Autodesk Fusion 360 part; units mm, degrees
sketch "Sketch1" plane through (0, 0, 0) normal (0, 0, 1) x (1, 0, 0)
  line L0 (0, 0) -> (76, 0)
  line L1 (76, 0) -> (76, 84)
  line L2 (76, 84) -> (0, 84)
  line L3 (0, 84) -> (0, 0)
  dimension "d1" = 76
  dimension "d2" = 84
extrude "Extrude1" add sketch "Sketch1" along normal blind 2.5
sketch "Sketch2" plane through (0, 0, 2.5) normal (0, 0, 1) x (-1, 0, 0)
  line L0 (0, -84) -> (0, 0)
  line L1 (0, 0) -> (-76, 0)
  line L2 (-76, 0) -> (-76, -84)
  line L3 (-76, -84) -> (0, -84)
  line L4 (0, -84) -> (-4, -84)
  line L5 (-4, -84) -> (-6, -84)
  line L6 (-6, -84) -> (-6, -69)
  line L7 (-6, -69) -> (-4, -69)
  line L8 (-4, -69) -> (-4, -84)
  line L9 (-4, -69) -> (-4, -51)
  line L10 (-4, -51) -> (-6, -51)
  line L11 (-6, -51) -> (-6, -33)
  line L12 (-6, -33) -> (-4, -33)
  line L13 (-4, -33) -> (-4, -51)
  line L14 (-4, -33) -> (-4, -15)
  line L15 (-4, -15) -> (-6, -15)
  line L16 (-6, -15) -> (-6, 0)
  line L17 (-6, 0) -> (-4, 0)
  line L18 (-4, 0) -> (-4, -15)
  line L19 (-6, -84) -> (-40, -84)
  line L20 (-4, -84) -> (-38, -84)
  line L21 (-38, -84) -> (-38, -65)
  line L22 (-72, -69) -> (-72, -84)
  line L23 (-70, -84) -> (-70, -69)
  line L24 (-72, -84) -> (-38, -84)
  line L25 (-70, -69) -> (-72, -69)
  line L26 (-72, -51) -> (-70, -51)
  line L27 (-70, -51) -> (-70, -33)
  line L28 (-72, -33) -> (-72, -51)
  line L29 (-70, -33) -> (-72, -33)
  line L30 (-72, -15) -> (-70, -15)
  line L31 (-70, -15) -> (-70, 0)
  line L32 (-72, 0) -> (-72, -15)
  line L33 (-70, 0) -> (-72, 0)
  dimension "d5" = 4
  dimension "d6" = 2
  dimension "d7" = 15
  dimension "d8" = 18
  dimension "d9" = 2
  dimension "d10" = 18
  dimension "d11" = 18
  dimension "d12" = 2
  dimension "d13" = 15
  dimension "d15" = 34
extrude "Extrude2" add sketch "Sketch2" along normal blind 3 contours L3 L5 L6 L7 L8 L20 | L1 L15 L16 L17 L18 | L10 L11 L12 L13 | L1 L30 L31 L32 L33 | L3 L22 L23 L24 L25 | L26 L27 L28 L29
sketch "Sketch3" plane through (0, 0, 2.5) normal (0, 0, 1) x (-1, 0, 0)
  line L0 (-72, -15) -> (-72, 0)
  line L1 (-72, 0) -> (-76, 0)
  line L2 (-76, 0) -> (-76, -84)
  line L3 (-76, -84) -> (-72, -84)
  line L4 (-72, -84) -> (-72, -69)
  line L5 (-72, -69) -> (-70, -69)
  line L6 (-70, -69) -> (-70, -84)
  line L7 (-70, -84) -> (-6, -84)
  line L8 (-6, -84) -> (-6, -69)
  line L9 (-6, -69) -> (-4, -69)
  line L10 (-4, -69) -> (-4, -84)
  line L11 (-4, -84) -> (0, -84)
  line L12 (0, -84) -> (0, 0)
  line L13 (0, 0) -> (-4, 0)
  line L14 (-4, 0) -> (-4, -15)
  line L15 (-4, -15) -> (-6, -15)
  line L16 (-6, -15) -> (-6, 0)
  line L17 (-6, 0) -> (-70, 0)
  line L18 (-70, 0) -> (-70, -15)
  line L19 (-70, -15) -> (-72, -15)
  line L20 (-4, -33) -> (-4, -51)
  line L21 (-4, -51) -> (-6, -51)
  line L22 (-6, -51) -> (-6, -33)
  line L23 (-6, -33) -> (-4, -33)
  line L24 (-70, -33) -> (-70, -51)
  line L25 (-70, -51) -> (-72, -51)
  line L26 (-72, -51) -> (-72, -33)
  line L27 (-72, -33) -> (-70, -33)
  line L28 (-70, -84) -> (-67.5, -84)
  line L29 (-67.5, -84) -> (-67.5, -79)
  line L30 (-67.5, -79) -> (-55.5, -79)
  line L31 (-55.5, -79) -> (-55.5, -77)
  line L32 (-55.5, -77) -> (-67.5, -77)
  line L33 (-67.5, -77) -> (-67.5, -79)
  line L34 (-67.5, -77) -> (-65.5, -77)
  line L35 (-65.5, -77) -> (-65.5, -67)
  line L36 (-65.5, -67) -> (-67.5, -67)
  line L37 (-67.5, -67) -> (-67.5, -77)
  line L38 (-67.5, -79) -> (-8.5, -79)
  line L39 (-8.5, -79) -> (-8.5, -76)
  line L40 (-8.5, -76) -> (-13.5, -76)
  line L41 (-13.5, -76) -> (-13.5, -74)
  line L42 (-13.5, -74) -> (-8.5, -74)
  line L43 (-8.5, -74) -> (-8.5, -76)
  line L44 (-8.5, -74) -> (-10.5, -74)
  line L45 (-10.5, -74) -> (-10.5, -64)
  line L46 (-10.5, -64) -> (-8.5, -64)
  line L47 (-8.5, -64) -> (-8.5, -74)
  line L48 (-67.5, -67) -> (-67.5, -16)
  line L49 (-67.5, -16) -> (-65.5, -16)
  line L50 (-65.5, -16) -> (-65.5, -6)
  line L51 (-65.5, -6) -> (-67.5, -6)
  line L52 (-67.5, -6) -> (-67.5, -16)
  line L53 (-65.5, -6) -> (-45.5, -6)
  line L54 (-45.5, -6) -> (-35.5, -6)
  line L55 (-35.5, -6) -> (-35.5, -8)
  line L56 (-35.5, -8) -> (-45.5, -8)
  line L57 (-45.5, -8) -> (-45.5, -6)
  line L58 (-35.5, -6) -> (-15.5, -6)
  line L59 (-15.5, -6) -> (-8.5, -6)
  line L60 (-8.5, -6) -> (-8.5, -8)
  line L61 (-8.5, -8) -> (-15.5, -8)
  line L62 (-15.5, -8) -> (-15.5, -6)
  line L63 (-8.5, -8) -> (-10.5, -8)
  line L64 (-10.5, -8) -> (-10.5, -18)
  line L65 (-10.5, -18) -> (-8.5, -18)
  line L66 (-8.5, -18) -> (-8.5, -8)
  dimension "d19" = 2.5
  dimension "d20" = 5
  dimension "d21" = 12
  dimension "d22" = 2
  dimension "d23" = 2
  dimension "d24" = 10
  dimension "d25" = 59
  dimension "d26" = 3
  dimension "d27" = 5
  dimension "d28" = 2
  dimension "d29" = 10
  dimension "d30" = 51
  dimension "d31" = 2
  dimension "d32" = 10
  dimension "d33" = 20
  dimension "d34" = 10
  dimension "d35" = 2
  dimension "d36" = 20
  dimension "d37" = 7
  dimension "d38" = 2
  dimension "d39" = 2
  dimension "d40" = 10
extrude "Extrude3" add sketch "Sketch3" along normal blind 5 contours L59 L60 L61 L62 L63 | L54 L55 L56 L57 | L49 L50 L51 L52 | L40 L41 L42 L43 L44 | L30 L31 L32 L33 L34 L38 | L32 L34 L35 L36 L37 | L42 L44 L45 L46 L47 | L61 L63 L64 L65 L66
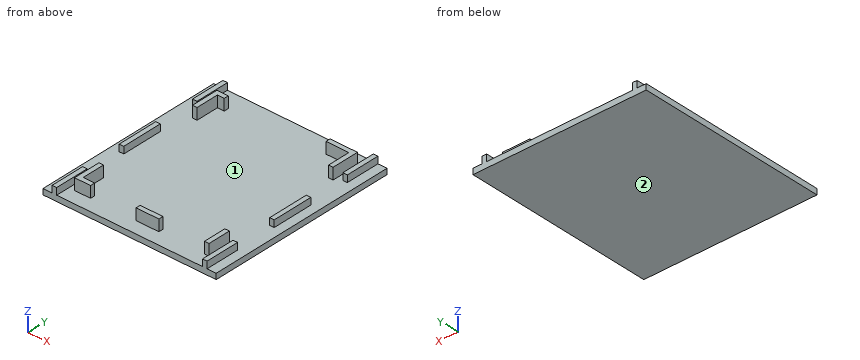
Geometry check sheet. Reference: the model listing, model coordinates, mm. Face numbers are marked on the shaded views. Round coordinates to 2 decimals unless told otherwise and drop trailing zeros. Loops run counter-clockwise (first coordinate to the right, second up) from the corner with the lowest first, then second, coordinate; pieces in that order, holes last. Notation, with made-up numbers: (82.25, 65.25) - (123.25, 65.25) arc R8 ccw to (123.25, 78.25) - close; hole circle Ø11 at (70, 77.25). An arc over 180 degrees is marked (long way). Write each question's results on one line, items separated by ' | '. Start each with the question number.
Q1. Cross-section at B-B on y = 43. Enter the section's corners in (x, z).
Q2. Cross-section at A-A on x = 71. Enter the section's corners in (y, z), and give its area (3 significant figures).
Q3. Cross-section at C-C on x = 60. Enter the section's corners in (y, z).
Q4. Gauge pin test, flat ends, axial feed: P1, Ø0.6, axis at x = 66.5, z = 4, coming from the +Y side; P2, Ø2, axis at x = 16, y = 14.5, coming from the +Z side; P3, Ø1.5, axis at y = 68, z = 4, coming from the +X side; P4, Ø3.5, axis at y = 6, z = 4, coming from the +X side. Record the tip position at first contact, or that the pin passes through.
Q5. Release check for a two-part mould opening along X. For the marked faces 1 and 2 record: +X half, -X half, draft (parallel to the pull), parting line (faces both ways), or undercut.
Q6. Thickness scan on line 1 (X direction, y = 7, z = 6.75); line 2 (X direction, y = 9, z = 5.75); line 3 (Y direction, x = 12, z = 7). Record the ranges inside material, lowest first. Write a range as [from, to].
Q7. Cross-section at D-D on y = 30.5. Enter the section's corners in (x, z), and give its area (3 significant figures).
Answers below:
1) outline: (0, 0) - (76, 0) - (76, 2.5) - (72, 2.5) - (72, 5.5) - (70, 5.5) - (70, 2.5) - (6, 2.5) - (6, 5.5) - (4, 5.5) - (4, 2.5) - (0, 2.5) - close
2) outline: (0, 0) - (84, 0) - (84, 5.5) - (69, 5.5) - (69, 2.5) - (51, 2.5) - (51, 5.5) - (33, 5.5) - (33, 2.5) - (15, 2.5) - (15, 5.5) - (0, 5.5) - close | area: 354 mm²
3) outline: (0, 0) - (84, 0) - (84, 2.5) - (79, 2.5) - (79, 7.5) - (77, 7.5) - (77, 2.5) - (0, 2.5) - close
4) P1: stops at y = 79 | P2: stops at z = 2.5 | P3: stops at x = 67.5 | P4: stops at x = 76
5) face 1: undercut | face 2: draft
6) line 1: x = [8.5, 15.5], [35.5, 45.5], [65.5, 67.5] | line 2: x = [8.5, 10.5], [65.5, 67.5] | line 3: y = [6, 8], [74, 76]
7) outline: (0, 0) - (76, 0) - (76, 2.5) - (0, 2.5) - close | area: 190 mm²
